Source: CAD feature listing. Evaluate the final solid. Frame: model axes, mm. A direction names the side the tool comes from. Round coordinates to 2 decimals unless told otherwise and drop trailing zeros. Order: outer loops, then holes, each group sorted by start corner. A loop starts at its lowest first (then second) coordinate and runs counter-clockwise, first axis right, second up. Notation, with made-up numbers: (71, 47) -> (96, 47) arc R15 ccw to (96, 69) -> close; hole circle Ø4 at (56, 24). An arc over 180 degrees is marked (long way). Answer as CSV lines item,"result". Start each with the question number.
(1) Contact query for flat-ended pins moving along their axis: P1, Ø8, axis at x = -9, z = -12, coming from the -Y side; P2, Ø1.5, axis at x = 10.5, y = 10.5, coming from the -Z side; P3, Ø3.5, axis at x = -10.5, y = -10.5, coming from the -Z side. Output: stop coordinate, or through.
(2) Set-up query: faces 1 (the flat face through (0, -21.15, 24)), 2 (the cylindrical face through (9.8, -9.34, -33.57)). Return all of +Z, -Z, +X, -X, +Y, -Y with unobstructed straight access to the full face (end or side cutting, diameter ignored); none if empty.
(3) Section query A-A (y = 0). Output: boundary loops of the cut face in (x, z), plus the area to 3 significant figures.
(4) Pull-direction query (X, two-part tool) for faces 3 (the flat face through (0, 0, 48.5)), 4 (the flat face through (11, -11, -28.5)), 5 (the cylindrical face through (0.867, -3.905, -48.36)); classes: +X half, -X half, draft (parallel to the pull), parting line (faces both ways), or undercut.
(5) Section query D-D (y = 16.5). Output: boundary loops of the cut face in (x, z).
(6) Line query: line 1 along Z through (x, y) = (19, 10); line 2 along Z through (x, y) = (4, 17.5); line 3 along Y through (x, z) = (-1.5, -4). Output: solid intervals per line, ascending. Write a range as from..to.
(7) Section query C-C (z = -19). Output: boundary loops of the cut face in (x, y).
```python
from build123d import *

# Parameters (mm, degrees)
SKETCH1_W           = 42.3
SKETCH1_H           = 42.3
BOSS_EXTRUDE1_DEPTH = 48.5
SKETCH3_R           = 18
BOSS_EXTRUDE2_DEPTH = 38.5
SKETCH5_R           = 4
BOSS_EXTRUDE3_DEPTH = 20
SKETCH6_R           = 1.5
CUT_EXTRUDE1_DEPTH  = 10


with BuildPart() as part:
    # Sketch1 → Boss-Extrude1 (new body)
    with BuildSketch(Plane.XY):
        Rectangle(SKETCH1_W, SKETCH1_H)
    extrude(amount=BOSS_EXTRUDE1_DEPTH)

    # Sketch3 → Boss-Extrude2 (add)
    with BuildSketch(Plane(origin=(0, 0, 0), x_dir=(-1, 0, 0), z_dir=(0, 0, -1))):
        Circle(SKETCH3_R)
    extrude(amount=BOSS_EXTRUDE2_DEPTH)

    # Sketch5 → Boss-Extrude3 (add)
    with BuildSketch(Plane(origin=(0, 0, -38.5), x_dir=(-1, 0, 0), z_dir=(0, 0, -1))):
        Circle(SKETCH5_R)
    extrude(amount=BOSS_EXTRUDE3_DEPTH)

    # Sketch6 → Cut-Extrude1 (cut)
    with BuildSketch(Plane(origin=(0, 0, -38.5), x_dir=(-1, 0, 0), z_dir=(0, 0, -1))):
        with Locations((-10.606601718, 10.606601718)):
            Circle(SKETCH6_R)
        with Locations((10.606601718, 10.606601718)):
            Circle(SKETCH6_R)
        with Locations((10.606601718, -10.606601718)):
            Circle(SKETCH6_R)
        with Locations((-10.606601718, -10.606601718)):
            Circle(SKETCH6_R)
    extrude(amount=-CUT_EXTRUDE1_DEPTH, mode=Mode.SUBTRACT)


solid = part.part
```
Answer block:
1,P1,"y = -17.29"
1,P2,"z = -28.5"
1,P3,"z = -38.5"
2,face 1,"+Z, -Z, +X, -X, -Y"
2,face 2,"-Z"
3,outline,"(-21.15, 0) -> (-18, 0) -> (-18, -38.5) -> (-4, -38.5) -> (-4, -58.5) -> (4, -58.5) -> (4, -38.5) -> (18, -38.5) -> (18, 0) -> (21.15, 0) -> (21.15, 48.5) -> (-21.15, 48.5) -> close"
3,area,"3,600 mm2"
4,face 3,"draft"
4,face 4,"undercut"
4,face 5,"parting line"
5,outline,"(-21.15, 0) -> (-7.19, 0) -> (-7.19, -38.5) -> (7.19, -38.5) -> (7.19, 0) -> (21.15, 0) -> (21.15, 48.5) -> (-21.15, 48.5) -> close"
6,line 1,"0..48.5"
6,line 2,"-38.5..48.5"
6,line 3,"-17.94..17.94"
7,outline,"circle Ø36 at (0, 0)"
